```python
from build123d import *

# Parameters (mm, degrees)
CROQUIS1_W              = 30
CROQUIS1_H              = 30
CROQUIS1_W_2            = 24
CROQUIS1_H_2            = 24
SALIENTE_EXTRUIR1_DEPTH = 130
REDONDEO2_R             = 2


with BuildPart() as part:
    # Croquis1 → Saliente-Extruir1 (new body)
    with BuildSketch(Plane(origin=(0, 0, 0), x_dir=(1, 0, 0), z_dir=(0, 1, 0))):
        Rectangle(CROQUIS1_W, CROQUIS1_H)
        Rectangle(CROQUIS1_W_2, CROQUIS1_H_2, mode=Mode.SUBTRACT)
    extrude(amount=SALIENTE_EXTRUIR1_DEPTH)

    # Redondeo2
    redondeo2_edges = [part.edges().sort_by_distance(p)[0] for p in [
        (-15, 130, 0),
        (0, 130, 15),
        (12, 65, 12),
        (-12, 65, 12),
        (15, 130, 0),
        (0, 0, 15),
        (-15, 0, 0),
        (0, 0, -15),
        (15, 0, 0),
        (0, 130, -15),
        (15, 65, 15),
        (-15, 65, 15),
        (-15, 65, -15),
        (15, 65, -15),
    ]]
    fillet(redondeo2_edges, radius=REDONDEO2_R)


solid = part.part
```
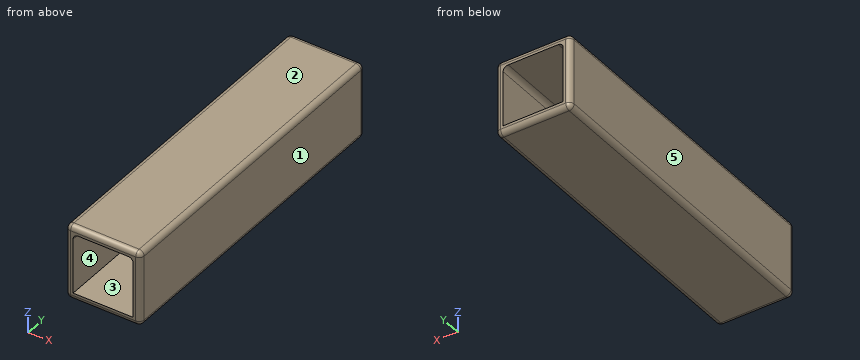
The listing builds one solid part. Answer for the finished solid, in the listing's coordinates (mm). Face numbers are marked on the shaded views. A direction names the side the tool comes from. Coordinates: 2 decimals unless noted, no trailing zeros. Loops run counter-clockwise (first coordinate to the right, second up) from the corner with the lowest first, then second, coordinate; pieces in that order, holes last. Notation, with made-up numbers: M 32.25,26 L 43.25,26 A20 cw 43.25,61 Z; hole C 7.5,78.25 d7. An arc over 180 degrees is marked long. Answer as CSV lines item,"result". Start each with the question number.
(1) Given pin 1 (1 mm diameter, centred on x = 10.5, z = 1.5, fed in from -Y), flat-ended and moving along its own axis, determine where the tip first touches the part or whether it passes through.
(2) The part is cut by section C-C (y = 90.5). Give the vertices of the cut face in (x, z).
(3) The part is cut by section B-B (x = 7.25). Give the vertices of the cut face in (y, z).
(4) The part is cut by section A-A (z = -8.5). Give the vertices of the cut face in (x, y).
(5) For the marked faces 4 and 5, determine the directions among +Z, -Z, +X, -X, +Y, -Y from which every point of the face is accessible in a straight line to the end or side of a thin tool.
(6) Find the intervals of material crossed by L1, parallel to Z at x = 10.25, y = 58; L2, parallel to X at y = 73, z = -2.25; L3, parallel to X at y = 74.5, z = 11, in increasing order. Write a range as [from, to].
(7) The mould has two halves that part along X. Classify the marked faces 1, 2 and 3: pulls with the +X half, pulls with the -X half, needs draft (parallel to the pull), parting line crosses it, or undercut.
Determined:
1,pin 1,"through"
2,outline,"M -15,-13 A2 ccw -13,-15 L 13,-15 A2 ccw 15,-13 L 15,13 A2 ccw 13,15 L -13,15 A2 ccw -15,13 Z; hole M -12,-12 L 12,-12 L 12,10 A2 ccw 10,12 L -10,12 A2 ccw -12,10 Z"
3,outline,"M 0,-13 A2 ccw 2,-15 L 128,-15 A2 ccw 130,-13 L 130,-12 L 0,-12 Z; M 0,12 L 130,12 L 130,13 A2 ccw 128,15 L 2,15 A2 ccw 0,13 Z"
4,outline,"M -15,2 A2 ccw -13,0 L -12,0 L -12,130 L -13,130 A2 ccw -15,128 Z; M 12,0 L 13,0 A2 ccw 15,2 L 15,128 A2 ccw 13,130 L 12,130 Z"
5,face 4,"+Y, -Y"
5,face 5,"+Z, -Z, -X, +Y, -Y"
6,L1,"[-15, -12], [11.98, 15]"
6,L2,"[-15, -12], [12, 15]"
6,L3,"[-15, -11.73], [11.73, 15]"
7,face 1,"pulls with the +X half"
7,face 2,"needs draft"
7,face 3,"undercut"
